The listing builds one solid part. Answer for the finished solid, in the listing's coordinates (mm). A direction names the side the tool comes from. Give positions to 0.01 mm unless a question says otherwise; leave off trailing zeros. Order: outer loops, then holes, each group sorted by start corner. A loop starts at its lowest first (then second) coordinate and runs counter-clockwise, first axis right, second up. Notation, with made-up numbers: (17, 80) - (72, 80) arc R14 ccw to (72, 104) - close; hole circle Ø10 at (9.5, 40.25). An arc over 180 degrees is marked (long way). Answer in a Markdown table with one row per item.
from build123d import *

# Parameters (mm, degrees)
CUT_EXTRUDE1_REACH      = 18.155
CUT_EXTRUDE1_END_RADIUS = 4.8
SKETCH2_R               = 1.505


with BuildPart() as part:
    # Sketch1 → Revolve1 (revolve)
    with BuildSketch(Plane.XY, mode=Mode.PRIVATE) as revolve1_sk:
        Polygon((2.955, 4), (2.955, 0), (4.8, 0), (4.8, 14.66), (3.3, 14.66), (3.3, 5.3), (0, 5.3), (0, 5), (1.515, 5), (1.515, 4), align=None)
    revolve(revolve1_sk.sketch.rotate(Axis((0, 0, 0), (0, 1, 0)), 90), axis=Axis((0, 0, 0), (0, 1, 0)))

    # Cut-Extrude1: up to this cylinder (the profile starts inside it)
    cut_extrude1_end = Plane(origin=(0, 10.803747, 0), z_dir=(0, -1, 0)) * Cylinder(CUT_EXTRUDE1_END_RADIUS, 46.91, mode=Mode.PRIVATE)
    # Sketch2 → Cut-Extrude1 (cut, up to the surface)
    with BuildSketch(Plane(origin=(0, 0, 0), x_dir=(0, 0, -1), z_dir=(1, 0, 0)), mode=Mode.PRIVATE) as cut_extrude1_sk1:
        with Locations((0, 10.803746972)):
            Circle(SKETCH2_R)
    cut_extrude1_tool1 = extrude(cut_extrude1_sk1.sketch, amount=-CUT_EXTRUDE1_REACH, mode=Mode.PRIVATE) & cut_extrude1_end
    add(cut_extrude1_tool1.solids().sort_by_distance((0, 10.803747, 0))[0], mode=Mode.SUBTRACT)


solid = part.part
Item 1: Which of the six approach directions +Z, -Z, +X, -X, +Y, -Y give full straight-line access (tool end or side, diameter ignored) to faces 4 (the face through (1.48, 4.49, 0.33)), 5 (the face through (0, 5.3, 0)), 6 (the face through (-3.859, 11.256, -1.436)), 7 (the face through (3.13, 0, -0.07))?
Answer block:
| item | result |
|---|---|
| face 4 | -Y |
| face 5 | +Y |
| face 6 | -X |
| face 7 | +Z, -Z, +X, -X, -Y |
Item 2: Find section B-B on x = 0. Write down the section's boundary in (y, z) (3 decimals).
Answer block:
| item | result |
|---|---|
| outline | (0, -4.8) - (14.66, -4.8) - (14.66, -3.3) - (5.3, -3.3) - (5.3, 3.3) - (14.66, 3.3) - (14.66, 4.8) - (0, 4.8) - (0, 2.955) - (4, 2.955) - (4, 1.515) - (5, 1.515) - (5, -1.515) - (4, -1.515) - (4, -2.955) - (0, -2.955) - close |
Item 3: Find section A-A on z = 0. Write down the section's boundary in (x, y) (3 decimals).
Answer block:
| item | result |
|---|---|
| outline | (-4.8, 0) - (-2.955, 0) - (-2.955, 4) - (-1.515, 4) - (-1.515, 5) - (1.515, 5) - (1.515, 4) - (2.955, 4) - (2.955, 0) - (4.8, 0) - (4.8, 14.66) - (3.3, 14.66) - (3.3, 5.3) - (-3.3, 5.3) - (-3.3, 9.299) - (-4.8, 9.299) - close; (-4.8, 12.309) - (-3.3, 12.309) - (-3.3, 14.66) - (-4.8, 14.66) - close |
Item 4: Find section C-C on y = 2. Write down the section's boundary in (x, z) (3 decimals).
Answer block:
| item | result |
|---|---|
| outline | circle Ø9.6 at (0, 0); hole circle Ø5.91 at (0, 0) |
Item 5: Each of these flat-tipped pins is pushed along its axis until it touches: P1, Ø5.5, axis at x = 0, z = 0, coming from the -Y side; P2, Ø1.8, axis at y = 10.8, z = 0, coming from the -X side; P3, Ø2, axis at y = 9.5, z = 1.5, coming from the -X side. Where does it stop, or does it pass through?
Answer block:
| item | result |
|---|---|
| P1 | y = 4 |
| P2 | x = 3.17 |
| P3 | x = -4.77 |
Item 6: Consider line 1 (X direction, y = 4.2, z = 0) (3 decimals); line 2 (X direction, y = 1.8, z = 0) (3 decimals); line 3 (Y direction, x = -4, z = 0). Determine where each line is inside the solid, lowest interval first.
Answer block:
| item | result |
|---|---|
| line 1 | -4.8 to -1.515, 1.515 to 4.8 |
| line 2 | -4.8 to -2.955, 2.955 to 4.8 |
| line 3 | 0 to 9.3, 12.31 to 14.66 |
Item 7: Determine the mould class of faces 1 (the face through (1.3, 4, 1.3)), 2 (the face through (4.686, 7.433, 1.041)), 3 (the face through (-3.3, 14.66, 1.1)) for opening direction X: pulls with the +X half, pulls with the -X half, needs draft (parallel to the pull), parting line crosses it, or undercut.
Answer block:
| item | result |
|---|---|
| face 1 | undercut |
| face 2 | parting line crosses it |
| face 3 | needs draft |
Item 8: Find section D-D on z = -2.75. Write down the section's boundary in (x, y), then the cut area to 3 significant figures.
Answer block:
| item | result |
|---|---|
| outline | (-3.93, 0) - (-1.08, 0) - (-1.08, 4) - (1.08, 4) - (1.08, 0) - (3.93, 0) - (3.93, 14.66) - (1.82, 14.66) - (1.82, 5.3) - (-1.82, 5.3) - (-1.82, 14.66) - (-3.93, 14.66) - close |
| area | 72.5 mm² |
